from build123d import *

# Parameters (mm, degrees)
SKETCH006_W      = 20
SKETCH006_H      = 20
EXTRUDE009_DEPTH = 15
EXTRUDE007_DEPTH = 135


with BuildPart() as extrude009:
    # Sketch006 (on Face2 of Extrude007) → Extrude009 (new body, symmetric)
    with BuildSketch(Plane(origin=(0, 0, 39), x_dir=(1, 0, 0), z_dir=(0, 0, -1))):
        with Locations((0, -231.482224)):
            Rectangle(SKETCH006_W, SKETCH006_H)
    extrude(amount=EXTRUDE009_DEPTH, both=True)


with BuildPart() as extrude009_1:
    # Extrude009 placement: moved
    add(extrude009.part.moved(Location((0, 0, 39))))


with BuildPart() as u067:
    # Sketch009 (on Face6 of Extrude006) → Extrude007 (new body)
    with BuildSketch(Plane(origin=(0, 136.482224, 0), x_dir=(-1, 0, 0), z_dir=(0, 1, 0))):
        Polygon((-32.5, 39), (-32.5, 81), (32.5, 81), (32.5, 39), (26.5, 39), (26.5, 75.5), (-26.5, 75.5), (-26.5, 39), align=None)
    extrude(amount=EXTRUDE007_DEPTH)

    # Cut002: cut Extrude009
    add(extrude009_1.part, mode=Mode.SUBTRACT)


solid = u067.part
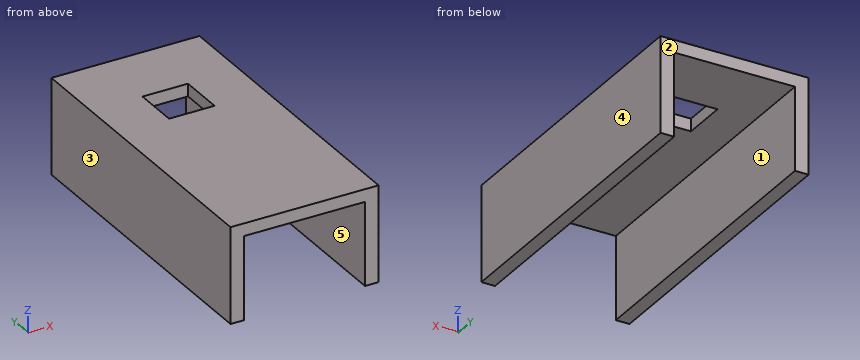
Verification items for the finished model (mm, model axes). Face numbers are marked on the shaded views. A direction names the side the tool comes from. Coordinates: 2 decimals unless noted, no trailing zeros. Order: outer loops, then holes, each group sorted by start corner. A loop starts at its lowest first (then second) coordinate and runs counter-clockwise, first axis right, second up. Notation, with made-up numbers: M -40,30 L -13,30 A18 cw -13,45 Z; hole C 66,61.25 d1. An arc over 180 degrees is marked long. One line per item, written item: value. Start each with the question number.
Item 1: Access from +Z, -Z, +X, -X, +Y, -Y to the whole of each face (thin tool, end or side, straight path). Record for the marked faces 4 and 5.
Item 2: Sectioned sample at A-A (y = 239). Enter the section's corners in (x, z), then the cut area to 4 significant figures.
Item 3: Gauge pin test, flat end, axial feed: pin 1 (1.5 mm diameter, centred on x = -1, y = 249, fed in from -Z). Record the tip position at first contact, or that the pin passes through.
Item 4: Scan lines: probe 1 along X at (y, z) = (203.5, 51); probe 2 along Z at (x, y) = (2.5, 176). Record each from-to range of solid material in increasing order.
Item 5: Sectioned sample at D-D (y = 189.5). Enter the section's corners in (x, z), then the cut area to 4 significant figures.
Item 6: Sectioned sample at B-B (z = 68.5). Enter the section's corners in (x, y).
Item 7: Sectioned sample at C-C (x = 3). Enter the section's corners in (y, z).
Item 8: Mould release check, pull along X, two halves, no side actions. Record for the marked faces 1, 2 and 3: released by +X, released by -X, zero draft, split by the parting line, or undercut.
Conclusion:
1. face 4: +Z, -Z, +X, +Y, -Y
1. face 5: -Z, +Y, -Y
2. outline: M -32.5,39 L -26.5,39 L -26.5,75.5 L -10,75.5 L -10,81 L -32.5,81 Z; M 10,75.5 L 26.5,75.5 L 26.5,39 L 32.5,39 L 32.5,81 L 10,81 Z
2. area: 685.5 mm^2
3. pin 1: stops at z = 75.5
4. probe 1: x = -32.5 to -26.5, 26.5 to 32.5
4. probe 2: z = 75.5 to 81
5. outline: M -32.5,39 L -26.5,39 L -26.5,75.5 L 26.5,75.5 L 26.5,39 L 32.5,39 L 32.5,81 L -32.5,81 Z
5. area: 795.5 mm^2
6. outline: M -32.5,136.48 L -26.5,136.48 L -26.5,271.48 L -32.5,271.48 Z; M 26.5,136.48 L 32.5,136.48 L 32.5,271.48 L 26.5,271.48 Z
7. outline: M 136.48,75.5 L 221.48,75.5 L 221.48,81 L 136.48,81 Z; M 241.48,75.5 L 271.48,75.5 L 271.48,81 L 241.48,81 Z
8. face 1: undercut
8. face 2: zero draft
8. face 3: released by -X
